Part model, mm, in its own coordinate system. Face numbers are marked on the shaded views. A direction names the side the tool comes from. Round coordinates to 2 decimals unless told otherwise and drop trailing zeros. Write each loop counter-clockwise with the first axis right and the second up, starting at its lowest first coordinate (ties: lowest second). Pieces come first, ordered by that corner, then holes. Notation, with made-up numbers: M 72,-34.75 L 118,-34.75 A17 cw 118,-29.75 Z; hole C -13,61 d10. An arc over 180 degrees is marked long. Answer as a JSON object with one key per item and string values. Group by question number.
1. Band-saw the part on B-B, the plane y = 87.5. Write the cut outline in (x, z), plus the area to 3 significant figures.
2. Band-saw the part on C-C, the plane y = 205.5. Write the cut outline in (x, z), plus the area to 3 significant figures.
3. Drop flat-ended pins along their axis: pin 1 (3 mm diameter, centred on y = 374, z = 58, fed in from -X); pin 2 (1 mm diameter, centred on y = 496, z = -214.5, fed in from +X); pin 3 (1.5 mm diameter, centred on x = 252.5, z = -15, fed in from -Y). Give the stop position or say it passes through.
4. Band-saw the part on A-A, the plane x = 0. Write the cut outline in (y, z), plus the area to 3 significant figures.
5. Which spindle directions (+Z, -Z, +X, -X, +Y, -Y) get a long thin tool onto all of the face, cutting with end or side? Do the marked faces 1 and 2. Say none if no direction does.
6. Drill centre lines: line 1 (Z direction, x = 0, y = 607); line 2 (Z direction, x = 0, y = 576.5); line 3 (Y direction, x = -33, z = 48.5). Where is each one in solid material? Low to high. Write a range as from..to.
from build123d import *

# Parameters (mm, degrees)
BOSS_EXTRUDE1_DEPTH      = 50.8
BOSS_EXTRUDE1_DEPTH_BACK = 50.8


with BuildPart() as part:
    # Sketch1 → Revolve1 (revolve)
    with BuildSketch(Plane.XY):
        Polygon((218.418109166, 505.968), (218.418109166, 649.224), (279.4, 649.224), (279.4, 598.424), (266.7, 598.424), (266.7, 617.474), (254, 617.474), (254, 598.424), (248.92, 598.424), (248.92, 486.918), (236.22, 486.918), (203.2, 0), (0, 0), (0, 19.05), (185.398109166, 19.05), align=None)
    revolve(axis=Axis((0, 19.05, 0), (0, -1, 0)))

    # Sketch2 → Boss-Extrude1 (add, two sides)
    with BuildSketch(Plane.XY) as boss_extrude1_sk:
        with BuildLine():
            Line((248.92, 509.524), (279.4, 488.181674235))
            ThreePointArc((279.4, 488.181674235), (299.197311316, 489.777633759), (301.333111503, 509.524))
            ThreePointArc((301.333111503, 509.524), (262.998722955, 546.823747439), (248.92, 598.424))
            Line((248.92, 598.424), (236.22, 598.424))
            Line((236.22, 598.424), (236.22, 518.416635735))
            Line((236.22, 518.416635735), (248.92, 509.524))
        make_face()
    extrude(amount=BOSS_EXTRUDE1_DEPTH)
    extrude(boss_extrude1_sk.sketch, amount=-BOSS_EXTRUDE1_DEPTH_BACK)


solid = part.part
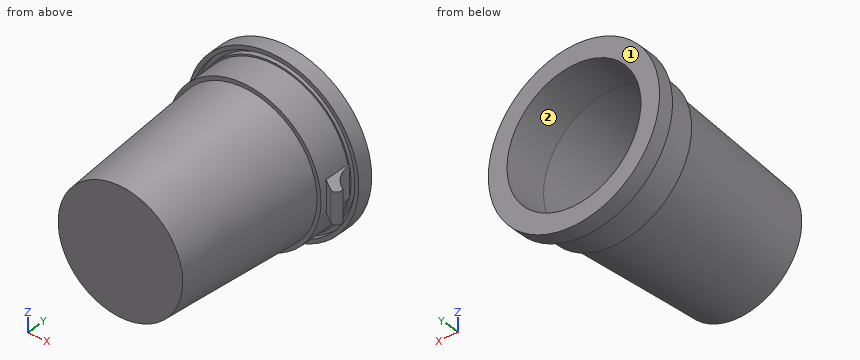
Worked answers:
{
 "1": {"outline": "C 0,0 d418.27; hole C 0,0 d380.08", "area": "23,900 mm^2"},
 "2": {"outline": "C 0,0 d434.27; hole C 0,0 d396.08", "area": "24,900 mm^2"},
 "3": {"pin 1": "stops at x = -221.48", "pin 2": "stops at x = 127.14", "pin 3": "stops at y = 506.49"},
 "4": {"outline": "M 0,-203.2 L 486.92,-236.22 L 486.92,-248.92 L 598.42,-248.92 L 598.42,-254 L 617.47,-254 L 617.47,-266.7 L 598.42,-266.7 L 598.42,-279.4 L 649.22,-279.4 L 649.22,-218.42 L 505.97,-218.42 L 19.05,-185.4 L 19.05,185.4 L 505.97,218.42 L 649.22,218.42 L 649.22,279.4 L 598.42,279.4 L 598.42,266.7 L 617.47,266.7 L 617.47,254 L 598.42,254 L 598.42,248.92 L 486.92,248.92 L 486.92,236.22 L 0,203.2 Z", "area": "38,200 mm^2"},
 "5": {"face 1": "+Z, -Z, +X, -X, +Y", "face 2": "+Y"},
 "6": {"line 1": "z = -279.4..-266.7, -254..-218.42, 218.42..254, 266.7..279.4", "line 2": "z = -248.92..-218.42, 218.42..248.92", "line 3": "y = 0..19.05"}
}
